Geometry: final body of the model. Coordinates: model frame, mm. Face numbers are marked on the shaded views. A direction names the side the tool comes from. Give positions to 0.01 mm unless a question says otherwise; leave off trailing zeros. Loops run counter-clockwise (first coordinate to the right, second up) from the corner with the lowest first, then second, coordinate; pieces in that order, holes last.
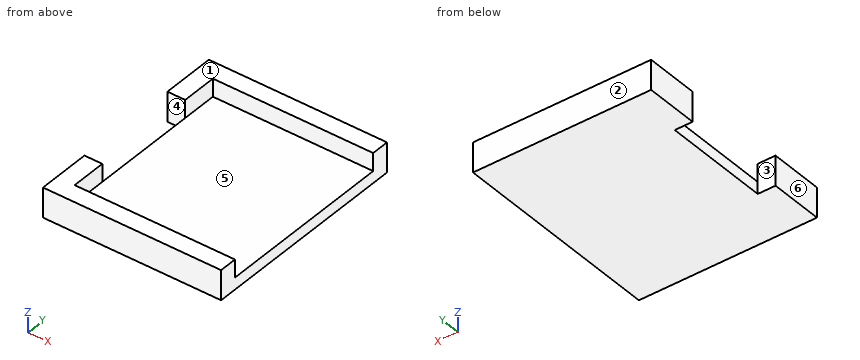
from build123d import *

# Parameters (mm, degrees)
SKETCH1_W           = 3
SKETCH1_H           = 6
SKETCH1_W_2         = 30
SKETCH1_H_2         = 3
BOSS_EXTRUDE1_DEPTH = 2
SKETCH1_3_W         = 3
SKETCH1_3_H         = 6
SKETCH1_3_W_2       = 30
SKETCH1_3_H_2       = 3
BOSS_EXTRUDE2_DEPTH = 5


with BuildPart() as part:
    # Sketch1 → Boss-Extrude1 (new body)
    with BuildSketch(Plane.XY):
        Polygon((-12, 15), (-12, 9), (-12, -9), (-12, -15), (15, -15), (15, 15), align=None)
        with Locations((-13.5, 12)):
            Rectangle(SKETCH1_W, SKETCH1_H)
        with Locations((-13.5, -12)):
            Rectangle(SKETCH1_W, SKETCH1_H)
        with Locations((0, 16.5)):
            Rectangle(SKETCH1_W_2, SKETCH1_H_2)
        with Locations((0, -16.5)):
            Rectangle(SKETCH1_W_2, SKETCH1_H_2)
    extrude(amount=BOSS_EXTRUDE1_DEPTH)

    # Sketch1_3 → Boss-Extrude2 (add)
    with BuildSketch(Plane.XY):
        with Locations((-13.5, 12)):
            Rectangle(SKETCH1_3_W, SKETCH1_3_H)
        with Locations((0, 16.5)):
            Rectangle(SKETCH1_3_W_2, SKETCH1_3_H_2)
        with Locations((-13.5, -12)):
            Rectangle(SKETCH1_3_W, SKETCH1_3_H)
        with Locations((0, -16.5)):
            Rectangle(SKETCH1_3_W_2, SKETCH1_3_H_2)
    extrude(amount=BOSS_EXTRUDE2_DEPTH)


solid = part.part
Item 1: Section query C-C on z = 1.1. Return loops of the section in (x, y), plus the area to 3 significant figures.
Values follow:
outline: (-15, -18) - (15, -18) - (15, 18) - (-15, 18) - (-15, 9) - (-12, 9) - (-12, -9) - (-15, -9) - close
area: 1,030 mm2
Item 2: Set-up query: the marked faces 4, 5 and 6. Return all of +Z, -Z, +X, -X, +Y, -Y with unobstructed straight access to the full face (end or side cutting, diameter ignored); none if empty.
Values follow:
face 4: +Z, -Z, -X
face 5: +Z, +X
face 6: +Z, -Z, -X, +Y, -Y
Item 3: Draft query along Y for the marked faces 1, 2 and 3. Return one class per face: +Y half, -Y half, draft (parallel to the pull), parting line (faces both ways), or undercut.
Values follow:
face 1: draft
face 2: +Y half
face 3: undercut
Item 4: Section query D-D on y = 10.5. Return loops of the section in (x, z), plus the area to 3 significant figures.
Values follow:
outline: (-15, 0) - (15, 0) - (15, 2) - (-12, 2) - (-12, 5) - (-15, 5) - close
area: 69.0 mm2
Item 5: Section query A-A on z = 2.9. Return loops of the section in (x, y), plus the area to 3 significant figures.
Values follow:
outline: (-15, -18) - (15, -18) - (15, -15) - (-12, -15) - (-12, -9) - (-15, -9) - close; (-15, 9) - (-12, 9) - (-12, 15) - (15, 15) - (15, 18) - (-15, 18) - close
area: 216 mm2
Item 6: Pin query (flat end, axial travel): pin 1 (1.5 mm diameter, centred on y = 6.5, z = 1, fed in from -X); pin 2 (0.9 mm diameter, centred on y = -13, z = 3.5, fed in from +X). Return the tip coordinate at first contact, or that it passes through.
Values follow:
pin 1: stops at x = -12
pin 2: stops at x = -12
Item 7: Ray query, probe 1 along Y at (x, z) = (-5.5, 4.35); probe 2 along Y at (x, z) = (-13.25, 4.7); probe 3 along X at (y, z) = (12.5, 2.95). Return the intervals inside material, ascending.
Values follow:
probe 1: y = -18 to -15, 15 to 18
probe 2: y = -18 to -9, 9 to 18
probe 3: x = -15 to -12
Item 8: Section query B-B on x = -0.5. Return loops of the section in (y, z), plus the area to 3 significant figures.
Values follow:
outline: (-18, 0) - (18, 0) - (18, 5) - (15, 5) - (15, 2) - (-15, 2) - (-15, 5) - (-18, 5) - close
area: 90.0 mm2
